Read the model definition and answer for the solid it produces. Units are mm, in the model's axes. Face numbers are marked on the shaded views. A direction names the side the tool comes from. Coordinates: 2 decimals unless noted, no trailing zeros. Write each loop counter-clockwise with the first axis right and the second up, starting at its lowest first coordinate (ties: lowest second). Pieces come first, ordered by that corner, then holes. Notation, with made-up numbers: (38, 82) -> (57, 82) arc R16 ccw to (57, 102) -> close; hole circle Ø10 at (80.25, 46.5). An arc over 180 degrees is marked (long way). Answer in a Markdown table with one row per item. Add a question column.
Item 1: Section C-C on y = 0 is taken. Count the separate pieces of the cut face and the enclosed holes in it, then the cut area to 3 significant figures.
Item 2: For a pull along X with two mould halves and no side action, classify the marked faces 3, 4 and 5 as +X half, -X half, draft (parallel to the pull), parting line (faces both ways), or undercut.
Item 3: Section A-A on z = 11.25 is taken. Write down the section's boundary in (x, y).
Item 4: Which of the six approach directions +Z, -Z, +X, -X, +Y, -Y give full straight-line access (tool end or side, diameter ignored) to the marked faces 1 and 2?
Item 5: Section B-B on x = -10 is taken. Write down the section's boundary in (y, z).
Item 6: Straight lines are drawn through the part: line 1 (Y direction, x = 10, z = 6.25); line 2 (X direction, y = -0.25, z = 17); line 3 (X direction, y = -1.25, z = 3.75). For each, find the intervals that lie inside material, in ascending order. Write a range as from..to.
Item 7: Given pin 1 Ø3.5 at (x, y) = (10, 0) entering from -Z; pin 2 Ø5.5 at (x, y) = (-10, 0) entering from +Z, each flat-ended and moving along its own axis, determine where each tip first touches the part or whether it passes through.
Autodesk Fusion 360 part; units mm, degrees
sketch "Sketch1" plane through (0, 0, 0) normal (0, 0, 1) x (1, 0, 0)
  line L0 (20, -10) -> (-20, -10)
  line L1 (-20, -10) -> (-20, 10)
  line L2 (-20, 10) -> (20, 10)
  line L3 (20, 10) -> (20, -10)
  line L4 (20, -10) -> (-20, 10) construction
  line L5 (-20, -10) -> (20, 10) construction
  line L6 (-20, 0) -> (20, 0) construction
  circle A0 centre (-10, 0) radius 1.7
  circle A1 centre (-10, 0) radius 3
  line L7 (0, 10) -> (0, -10) construction
  circle A2 centre (10, 0) radius 1.7
  circle A3 centre (10, 0) radius 3
  line L8 (-6.1906, 3.4245) -> (-13.346, 7.0022)
  line L9 (-13.346, 7.0022) -> (-12.8094, 8.0755)
  line L10 (-12.8094, 8.0755) -> (-5.654, 4.4978)
  line L11 (-5.654, 4.4978) -> (-6.1906, 3.4245)
  line L12 (-6.1906, 3.4245) -> (-12.8094, 8.0755) construction
  line L13 (-13.346, 7.0022) -> (-5.654, 4.4978) construction
  line L14 (6.1906, 3.4245) -> (13.346, 7.0022)
  line L15 (13.346, 7.0022) -> (12.8094, 8.0755)
  line L16 (12.8094, 8.0755) -> (5.654, 4.4978)
  line L17 (5.654, 4.4978) -> (6.1906, 3.4245)
  line L18 (-13.0094, 7.6755) -> (-12.0094, 7.6755)
  line L19 (13.0094, 7.6755) -> (12.0094, 7.6755)
  point P0 (-9.5, 5.75)
  dimension "d1" = 40
  dimension "d2" = 20
  dimension "d3" = 3.4
  dimension "d4" = 6
  dimension "d5" = 10
  dimension "d17" = 8
  dimension "d18" = 1.2
  dimension "d19" = 9.5
  dimension "d20" = 4.25
  dimension "d24" = 0.4
extrude "Extrude1" add sketch "Sketch1" along normal blind 18 contours L0 L1 L2 L3 | A1 | A3 | L8 L9 L10 L11 L18 | L9 L10 L18 | L14 L15 L16 L17 L19 | L15 L16 L19
extrude "Extrude2" cut sketch "Sketch1" against normal blind 3 from surface at 18 contours A1 | A3
fillet "Fillet1" radius 3 4 edges at (-20, 10, 9) (-20, -10, 9) (20, -10, 9) (20, 10, 9)
chamfer "Chamfer1" distance 1 angle 45 8 edges at (0, 10, 18) (-19.1213, 9.1213, 18) (-20, 0, 18) (-19.1213, -9.1213, 18) (0, -10, 18) (19.1213, -9.1213, 18) (20, 0, 18) (19.1213, 9.1213, 18)
chamfer "Chamfer2" distance 0.4 angle 45 10 edges at (7.203, 1.0848, 18) (-12.797, 1.0848, 18) (0, -10, 0) (-19.1213, -9.1213, 0) (-20, 0, 0) (-19.1213, 9.1213, 0) (0, 10, 0) (19.1213, 9.1213, 0) (20, 0, 0) (19.1213, -9.1213, 0)
chamfer "Chamfer3" distance 0.2 angle 45 2 edges at (-11.585, -0.6147, 15) (8.415, -0.6147, 15)
chamfer "Chamfer4" distance 0.4 angle 45 2 edges at (-11.585, 0.6147, 0) (8.415, 0.6147, 0)
extrude "Extrude3" cut sketch "Sketch1" against normal blind 0.8 from surface at 18 contours L8 L9 L10 L11 L18 | L14 L15 L16 L17 L19
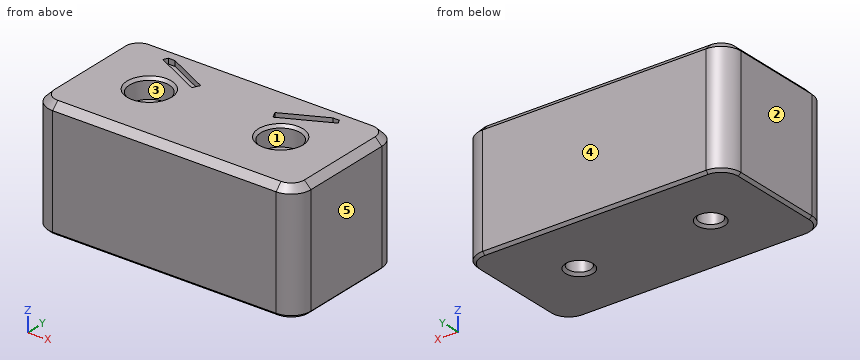
Results below:
| question | item | result |
|---|---|---|
| 1 | separate pieces | 3 |
| 1 | enclosed holes | 0 |
| 1 | area | 580 mm2 |
| 2 | face 3 | undercut |
| 2 | face 4 | draft |
| 2 | face 5 | +X half |
| 3 | outline | (-20, -7) arc R3 ccw to (-17, -10) -> (17, -10) arc R3 ccw to (20, -7) -> (20, 7) arc R3 ccw to (17, 10) -> (-17, 10) arc R3 ccw to (-20, 7) -> close; hole circle Ø3.4 at (-10, 0); hole circle Ø3.4 at (10, 0) |
| 4 | face 1 | +Z |
| 4 | face 2 | +Z, -Z, -X, +Y, -Y |
| 5 | outline | (-10, 0.4) -> (-9.6, 0) -> (-2.1, 0) -> (-1.7, 0.4) -> (-1.7, 14.8) -> (-1.9, 15) -> (-3, 15) -> (-3, 17.6) -> (-3.4, 18) -> (-9, 18) -> (-10, 17) -> close; (1.7, 0.4) -> (2.1, 0) -> (9.6, 0) -> (10, 0.4) -> (10, 17) -> (9, 18) -> (6.67, 18) -> (6.67, 17.2) -> (5.33, 17.2) -> (5.33, 18) -> (3.4, 18) -> (3, 17.6) -> (3, 15) -> (1.9, 15) -> (1.7, 14.8) -> close |
| 6 | line 1 | y = -10..-1.7, 1.7..10 |
| 6 | line 2 | x = -20..-12.99, -7.01..7.01, 12.99..20 |
| 6 | line 3 | x = -20..-11.15, -8.85..8.85, 11.15..20 |
| 7 | pin 1 | stops at z = 0.35 |
| 7 | pin 2 | stops at z = 15 |
